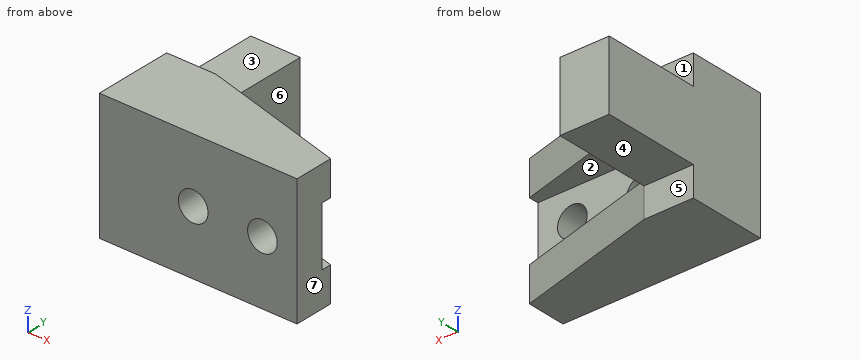
from build123d import *

# Parameters (mm, degrees)
EXTRUDE_1_DEPTH     = 13
SKETCH_2_W          = 3
SKETCH_2_H          = 10
CUT_EXTRUDE_1_DEPTH = 30.883105595
CUT_EXTRUDE_2_DEPTH = 5
SKETCH_4_R          = 1.5
CUT_EXTRUDE_3_DEPTH = 29.178005607


with BuildPart() as part:
    # 草图1 → 凸台-拉伸1 (new body)
    with BuildSketch(Plane.XY):
        Polygon((0, 0), (20, 0), (20, 4), (5, 8), (5, 18), (0, 18), align=None)
    extrude(amount=EXTRUDE_1_DEPTH)

    # 草图2 → 切除-拉伸1 (cut, through all)
    with BuildSketch(Plane.ZY):
        with Locations((1.5, 13)):
            Rectangle(SKETCH_2_W, SKETCH_2_H)
        with Locations((11.5, 13)):
            Rectangle(SKETCH_2_W, SKETCH_2_H)
    extrude(amount=-CUT_EXTRUDE_1_DEPTH, mode=Mode.SUBTRACT)

    # 草图3 → 切除-拉伸2 (cut)
    with BuildSketch(Plane(origin=(0, 8, 0), x_dir=(-1, 0, 0), z_dir=(0, -1, 0))):
        Polygon((-5, -6.5), (-5, -9.5), (-20, -9.5), (-20, -3.5), (-5, -3.5), align=None)
    extrude(amount=CUT_EXTRUDE_2_DEPTH, mode=Mode.SUBTRACT)

    # 草图4 → 切除-拉伸3 (cut, through all)
    with BuildSketch(Plane(origin=(0, 3, 0), x_dir=(1, 0, 0), z_dir=(0, 1, 0))):
        with Locations(Location((16.5, -6.5, 0), (0, 0, 270))):
            Circle(SKETCH_4_R)
        with Locations(Location((9.5, -6.5, 0), (0, 0, 270))):
            Circle(SKETCH_4_R)
    extrude(amount=-CUT_EXTRUDE_3_DEPTH, mode=Mode.SUBTRACT)


solid = part.part
Input: part model. Units: mm. Frame: model coordinates. Face numbers are marked on the shaded views. A direction names the side the tool comes from. Coordinates: 2 decimals unless noted, no trailing zeros. Loops run counter-clockwise (first coordinate to the right, second up) from the corner with the lowest first, then second, coordinate; pieces in that order, holes last. Notation, with made-up numbers: (-34, -16) -> (24, -16) arc R24 cw to (24, 14) -> close; hole circle Ø8 at (41.25, 56). An arc over 180 degrees is marked (long way). Write item = value, one per line. Start each with the question number.
Item 1: Mould query, pull axis Z, two halves, no side actions, for the marked faces 1, 2, 3 and 4. Classes: pulls with the +Z half, pulls with the -Z half, needs draft (parallel to the pull), parting line crosses it, or undercut.
Item 2: Cut plane D-D, the plane z = 9.25. Return loops of the section in (x, y).
Item 3: Reachability of the marked faces 5, 6 and 7 from +Z, -Z, +X, -X, +Y, -Y: full face, straight path, thin tool, end or side. Return the list, or none.
Item 4: Cut plane A-A, the plane x = 9.5. Return loops of the section in (y, z).
Item 5: Material intervals for line 1 (X direction, y = 1.45, z = 6.5); line 2 (X direction, y = 13.25, z = 3.75); line 3 (Z direction, x = 11, y = 3.25), sorted ascending.
Item 6: Cut plane C-C, the plane x = 12.5. Return loops of the section in (y, z).
Item 7: First-contact query: P1, Ø1.5, axis at x = 2, z = 12, coming from the +Y side; P2, Ø1.5, axis at x = 9.5, z = 9.5, coming from the -Y side; P3, Ø1.5, axis at x = 3.5, y = 13.5, coming from the +Z side; P4, Ø1.5, axis at x = 1.5, y = 14.5, coming from the -Z side. Flat tips, straight axial feed; report the tip coordinate or a pass-through.
Item 8: Cut plane B-B, the plane z = 6.5. Return loops of the section in (x, y).
Ans:
q1.face_1 = needs draft
q1.face_2 = undercut
q1.face_3 = pulls with the +Z half
q1.face_4 = pulls with the -Z half
q2.outline = (0, 0) -> (20, 0) -> (20, 3) -> (5, 3) -> (5, 18) -> (0, 18) -> close
q3.face_5 = -Z, +X, -X, +Y
q3.face_6 = +X, +Y
q3.face_7 = +Z, -Z, +X, +Y, -Y
q4.outline = (0, 0) -> (6.8, 0) -> (6.8, 3.5) -> (3, 3.5) -> (3, 5) -> (0, 5) -> close; (0, 8) -> (3, 8) -> (3, 9.5) -> (6.8, 9.5) -> (6.8, 13) -> (0, 13) -> close
q5.line_1 = 0 to 8, 11 to 15, 18 to 20
q5.line_2 = 0 to 5
q5.line_3 = 0 to 3.5, 9.5 to 13
q6.outline = (0, 0) -> (6, 0) -> (6, 3.5) -> (3, 3.5) -> (3, 9.5) -> (6, 9.5) -> (6, 13) -> (0, 13) -> close
q7.P1 = 8
q7.P2 = 0
q7.P3 = 10
q7.P4 = 3
q8.outline = (0, 0) -> (8, 0) -> (8, 3) -> (5, 3) -> (5, 18) -> (0, 18) -> close; (11, 0) -> (15, 0) -> (15, 3) -> (11, 3) -> close; (18, 0) -> (20, 0) -> (20, 3) -> (18, 3) -> close
